from build123d import *

# Parameters (mm, degrees)
ESQUISSE1_R             = 2
ESQUISSE1_R_2           = 1.5
BASE_EXTRUSION_DEPTH    = 8
ENL_V_MAT_EXTRU_1_DEPTH = 24
ENL_V_MAT_EXTRU_2_DEPTH = 3
BOSS_EXTRU_2_DEPTH      = 0.75
ENL_V_MAT_EXTRU_3_DEPTH = 5.75
CONG_1_R                = 0.5
ESQUISSE9_R             = 3
BOSS_EXTRU_3_DEPTH      = 1
ESQUISSE10_R            = 1.25
ENL_V_MAT_EXTRU_4_DEPTH = 8


with BuildPart() as part:
    # Esquisse1 → Base-Extrusion (new body)
    with BuildSketch(Plane.XY):
        with BuildLine():
            Line((0, 4), (29, 4))
            ThreePointArc((29, 4), (33, 0), (29, -4))
            Line((29, -4), (0, -4))
            ThreePointArc((0, -4), (-4, 0), (0, 4))
        make_face()
        with Locations((29, 0)):
            Circle(ESQUISSE1_R, mode=Mode.SUBTRACT)
        with Locations((16.5, 0)):
            Circle(ESQUISSE1_R_2, mode=Mode.SUBTRACT)
    extrude(amount=BASE_EXTRUSION_DEPTH)

    # Esquisse2 → Enlèv. mat.-Extru.1 (cut, symmetric)
    with BuildSketch(Plane(origin=(0, 0, 0), x_dir=(1, 0, 0), z_dir=(0, 1, 0))):
        Polygon((-4, 0), (5, 0), (24, -2), (32, -2), (34, -2), (34, 2), (-5, 2), (-5, 0), align=None)
        Polygon((30, -8), (24, -8), (5, -6), (-5, -6), (-5, -9), (35, -9), (35, -8), align=None)
    extrude(amount=ENL_V_MAT_EXTRU_1_DEPTH, both=True, mode=Mode.SUBTRACT)

    # Esquisse3 → Enlèv. mat.-Extru.2 (cut)
    with BuildSketch(Plane.XY.offset(8)):
        with BuildLine():
            Line((26.143442915, 2.846006946), (19.097354695, 2.846006946))
            ThreePointArc((19.097354695, 2.846006946), (18.640423669, 2.549019353), (18.726304024, 2.010863096))
            ThreePointArc((18.726304024, 2.010863096), (19.5, 0), (18.726304024, -2.010863096))
            ThreePointArc((18.726304024, -2.010863096), (18.640423669, -2.549019353), (19.097354695, -2.846006946))
            Line((19.097354695, -2.846006946), (26.143442915, -2.846006946))
            ThreePointArc((26.143442915, -2.846006946), (26.595475356, -2.559704564), (26.529835939, -2.028673634))
            ThreePointArc((26.529835939, -2.028673634), (25.80356023, 0), (26.529835939, 2.028673634))
            ThreePointArc((26.529835939, 2.028673634), (26.595475356, 2.559704564), (26.143442915, 2.846006946))
        make_face()
        with BuildLine():
            Line((13.902645305, 2.846006946), (3.239791878, 2.846006946))
            ThreePointArc((3.239791878, 2.846006946), (2.794468717, 2.573355319), (2.834817893, 2.052756078))
            ThreePointArc((2.834817893, 2.052756078), (3.5, 0), (2.834817893, -2.052756078))
            ThreePointArc((2.834817893, -2.052756078), (2.794468717, -2.573355319), (3.239791878, -2.846006946))
            Line((3.239791878, -2.846006946), (13.902645305, -2.846006946))
            ThreePointArc((13.902645305, -2.846006946), (14.359576331, -2.549019353), (14.273695976, -2.010863096))
            ThreePointArc((14.273695976, -2.010863096), (13.5, 0), (14.273695976, 2.010863096))
            ThreePointArc((14.273695976, 2.010863096), (14.359576331, 2.549019353), (13.902645305, 2.846006946))
        make_face()
    enl_v_mat_extru_2 = extrude(amount=-ENL_V_MAT_EXTRU_2_DEPTH, mode=Mode.SUBTRACT)

    # Symétrie1: Enlèv. mat.-Extru.2 across plane
    add(enl_v_mat_extru_2.mirror(Plane(origin=(0, 0, 4), x_dir=(1, 0, 0), z_dir=(0, 0, -1))), mode=Mode.SUBTRACT)

    # Esquisse7 → Boss.-Extru.2 (add)
    with BuildSketch(Plane.XZ.offset(4)):
        Polygon((5, 3.25), (24, 3.25), (29, 4), (24, 4.75), (5, 4.75), (0, 4), align=None)
    boss_extru_2 = extrude(amount=BOSS_EXTRU_2_DEPTH)

    # Symétrie2: Boss.-Extru.2 across plane
    add(boss_extru_2.mirror(Plane.ZX))

    # Esquisse8 → Enlèv. mat.-Extru.3 (cut, through all)
    with BuildSketch(Plane.XY.offset(4.75)):
        Polygon((0, 4), (5, 4.75), (5, 7), (0, 7), align=None)
        Polygon((24, 4.75), (29, 4), (29, 7), (24, 7), align=None)
        Polygon((29, -7), (24, -7), (24, -4.75), (29, -4), align=None)
        Polygon((5, -4.75), (5, -7), (0, -7), (0, -4), align=None)
    extrude(amount=-ENL_V_MAT_EXTRU_3_DEPTH, mode=Mode.SUBTRACT)

    # Congé1
    cong_1_edges = [part.edges().sort_by_distance(p)[0] for p in [
        (26.5, -4, 2),
        (14.5, -4, 1),
        (2.5, -4, 0),
        (33, 0, 2),
        (33, 0, 8),
        (26.5, -4, 8),
        (14.5, -4, 7),
        (2.5, -4, 6),
        (2.5, 4, 6),
        (-4, 0, 6),
        (14.5, 4, 7),
        (26.5, 4, 8),
        (2.5, 4, 0),
        (14.5, 4, 1),
        (26.5, 4, 2),
        (-4, 0, 0),
    ]]
    fillet(cong_1_edges, radius=CONG_1_R)

    # Esquisse9 → Boss.-Extru.3 (add)
    with BuildSketch(Plane.XY.offset(6)):
        Circle(ESQUISSE9_R)
    extrude(amount=BOSS_EXTRU_3_DEPTH)

    # Esquisse10 → Enlèv. mat.-Extru.4 (cut, through all)
    with BuildSketch(Plane.XY.offset(7)):
        Circle(ESQUISSE10_R)
    extrude(amount=-ENL_V_MAT_EXTRU_4_DEPTH, mode=Mode.SUBTRACT)


solid = part.part
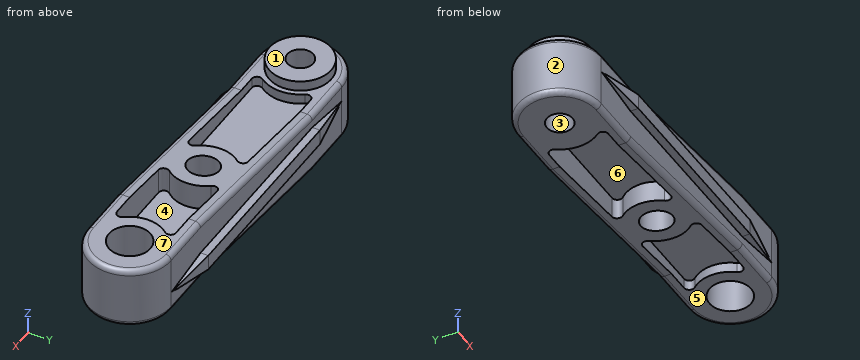
Verification items for the finished model (mm, model axes). Face numbers are marked on the shaded views. A direction names the side the tool comes from. Coordinates: 2 decimals unless noted, no trailing zeros. One line per item, written item: value. Start each with the question number.
Item 1: Mould release check, pull along Y, two halves, no side actions. Record for the marked faces 1, 2 and 3: released by +Y, released by -Y, zero draft, split by the parting line, or undercut.
Item 2: Sectioned sample at A-A (z = 6.5). Count the separate pieces of the cut face and the enclosed holes in it, then the cut area to 3 significant figures.
Item 3: Scan lines: probe 1 along Y at (x, z) = (11, 2); probe 2 along Y at (x, z) = (16.5, 4); probe 3 along Y at (x, z) = (14, 1). Record each from-to range of solid material in increasing order.
Item 4: Gauge pin test, flat ends, axial feed: pin 1 (1 mm diameter, centred on x = 15, z = 6, fed in from +Y); pin 2 (1.7 mm diameter, centred on x = 21.5, y = 1, fed in from +Z); pin 3 (1.7 mm diameter, centred on x = 21.5, z = 2, fed in from -Y); pin 4 (3 mm diameter, centred on x = 29, y = 0, fed in from +Z). Record the tip position at first contact, or that the pin passes through.
Item 5: Access from +Z, -Z, +X, -X, +Y, -Y to the whole of each face (thin tool, end or side, straight path). Record for the marked faces 4, 5, 6 and 7.
Conclusion:
1. face 1: zero draft
1. face 2: split by the parting line
1. face 3: undercut
2. separate pieces: 2
2. enclosed holes: 4
2. area: 118 mm^2
3. probe 1: y = -4 to -2.85, 2.85 to 4
3. probe 2: y = -4.75 to -1.5, 1.5 to 4.75
3. probe 3: y = -3.72 to -2.84, -1.66 to 1.66, 2.84 to 3.72
4. pin 1: stops at y = 4
4. pin 2: stops at z = 5
4. pin 3: stops at y = -4
4. pin 4: passes through
5. face 4: +Z
5. face 5: -Z, +X, +Y, -Y
5. face 6: -Z
5. face 7: +Z, +X, -X, +Y, -Y
